Here's how the part is built. I have some questions about the finished solid (model axes, mm). Face numbers are marked on the shaded views. Round coordinates to 2 decimals unless told otherwise and drop trailing zeros. Write each loop counter-clockwise with the first axis right and the second up, starting at its lowest first coordinate (ties: lowest second). Pieces come first, ordered by that corner, then holes. Notation, with made-up numbers: (62, 12.25) -> (114, 12.25) arc R31 ccw to (114, 50.25) -> close; hole circle Ø7 at (69, -39). An arc over 180 degrees is marked (long way). Answer as CSV lines item,"result".
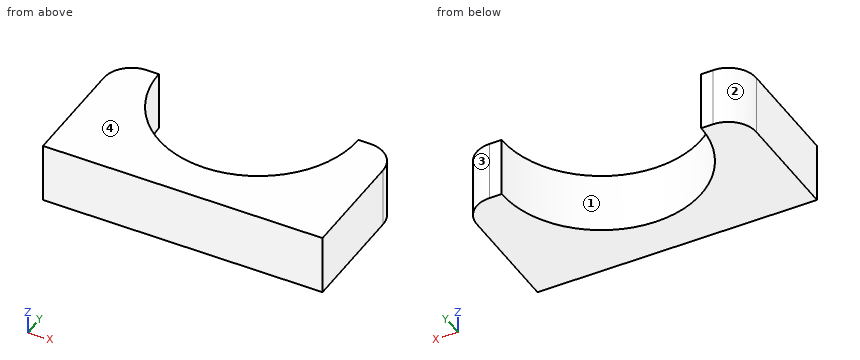
from build123d import *

# Parameters (mm, degrees)
BOSS_EXTRUDE1_DEPTH = 7.5
FILLET1_R           = 3.5


with BuildPart() as part:
    # Sketch1 → Boss-Extrude1 (new body)
    with BuildSketch(Plane.XY):
        with BuildLine():
            Line((-17.5, 0), (17.5, 0))
            Line((17.5, 0), (17.5, 17.5))
            Line((17.5, 17.5), (12.5, 17.5))
            ThreePointArc((12.5, 17.5), (0, 5), (-12.5, 17.5))
            Line((-12.5, 17.5), (-17.5, 17.5))
            Line((-17.5, 17.5), (-17.5, 0))
        make_face()
    extrude(amount=BOSS_EXTRUDE1_DEPTH)

    # Fillet1
    fillet1_edges = [part.edges().sort_by_distance(p)[0] for p in [
        (-17.5, 17.5, 3.75),
        (17.5, 17.5, 3.75),
    ]]
    fillet(fillet1_edges, radius=FILLET1_R)


solid = part.part
Item 1: Suppose I cut it at C-C, the plane x = -3.5. List the corners of the cut face in (y, z) for me, then the cut area to 4 significant figures.
Results found:
outline,"(0, 0) -> (5.5, 0) -> (5.5, 7.5) -> (0, 7.5) -> close"
area,"41.25 mm²"
Item 2: Suppose I cut it at A-A, the plane z = 0.75. List the corners of the cut face in (x, y) for me.
Results found:
outline,"(-17.5, 0) -> (17.5, 0) -> (17.5, 14) arc R3.5 ccw to (14, 17.5) -> (12.5, 17.5) arc R12.5 cw to (-12.5, 17.5) -> (-14, 17.5) arc R3.5 ccw to (-17.5, 14) -> close"
Item 3: Suppose I cut it at B-B, the plane y = 15.5. List the corners of the cut face in (x, z) for me.
Results found:
outline,"(-17.16, 0) -> (-12.34, 0) -> (-12.34, 7.5) -> (-17.16, 7.5) -> close; (12.34, 0) -> (17.16, 0) -> (17.16, 7.5) -> (12.34, 7.5) -> close"
Item 4: I need wall thicknesses on L1, parallel to X at y = 9.25, z = 3.5; L2, parallel to X at y = 10, z = 2.75; L3, parallel to Y at x = -7, z = 3. Which ranges of each line are inside material? Lowest first, please.
Results found:
L1,"x = -17.5 to -9.39, 9.39 to 17.5"
L2,"x = -17.5 to -10, 10 to 17.5"
L3,"y = 0 to 7.14"
Item 5: Suppose I cut it at D-D, the plane y = 9.25. List the corners of the cut face in (x, z) for me, then the cut area to 3 significant figures.
Results found:
outline,"(-17.5, 0) -> (-9.39, 0) -> (-9.39, 7.5) -> (-17.5, 7.5) -> close; (9.39, 0) -> (17.5, 0) -> (17.5, 7.5) -> (9.39, 7.5) -> close"
area,"122 mm²"
Item 6: If we mould it in two halves opening along X, with no side actions, what happens to the marked faces 1, 2, 3 and 4? For each: pulls with the +X half, pulls with the -X half, needs draft (parallel to the pull), parting line crosses it, or undercut.
Results found:
face 1,"undercut"
face 2,"pulls with the -X half"
face 3,"pulls with the +X half"
face 4,"needs draft"
